The listing builds one solid part. Answer for the finished solid, in the listing's coordinates (mm). A direction names the side the tool comes from. Coordinates: 2 decimals unless noted, no trailing zeros. Order: outer loops, then holes, each group sorted by start corner. A loop starts at its lowest first (then second) coordinate and runs counter-clockwise, first axis right, second up. Notation, with made-up numbers: (74, 81) - (82, 81) arc R13 ccw to (82, 96) - close; hole circle Ø3 at (32.25, 40). An arc over 180 degrees is marked (long way). One line per item, written item: value. Start each with the question number.
```python
from build123d import *

# Parameters (mm, degrees)
SKETCH1_R           = 2
SKETCH1_R_2         = 6
SKETCH1_R_3         = 1.5
BOSS_EXTRUDE1_DEPTH = 3


with BuildPart() as part:
    # Sketch1 → Boss-Extrude1 (new body)
    with BuildSketch(Plane.XY):
        with BuildLine():
            Line((-12.06516619, -3.534722735), (-7.905685951, -9.775614029))
            ThreePointArc((-7.905685951, -9.775614029), (-8.460728899, -12.549046438), (-11.234161307, -11.99400349))
            Line((-11.234161307, -11.99400349), (-11.927408014, -10.953854941))
            ThreePointArc((-11.927408014, -10.953854941), (-12.563289537, -10.527895875), (-13.314124218, -10.676333467))
            Line((-13.314124218, -10.676333467), (-14.001074492, -11.1341777))
            ThreePointArc((-14.001074492, -11.1341777), (-14.438315509, -11.838795077), (-14.193503634, -12.631090792))
            ThreePointArc((-14.193503634, -12.631090792), (15.810257944, 10.537349939), (-17.120545284, -8.239352474))
            ThreePointArc((-17.120545284, -8.239352474), (-16.483484999, -8.770219263), (-15.664866588, -8.637821183))
            Line((-15.664866588, -8.637821183), (-14.977916314, -8.17997695))
            ThreePointArc((-14.977916314, -8.17997695), (-14.551957247, -7.544095427), (-14.70039484, -6.793260745))
            Line((-14.70039484, -6.793260745), (-15.393641546, -5.753112196))
            ThreePointArc((-15.393641546, -5.753112196), (-14.838598598, -2.979679788), (-12.06516619, -3.534722735))
        make_face()
        with Locations((-8.873557843, 13.313901427)):
            Circle(SKETCH1_R, mode=Mode.SUBTRACT)
        with Locations((13.31390139, 8.873557851)):
            Circle(SKETCH1_R, mode=Mode.SUBTRACT)
        with Locations((8.873557814, -13.313901383)):
            Circle(SKETCH1_R, mode=Mode.SUBTRACT)
        Circle(SKETCH1_R_2, mode=Mode.SUBTRACT)
        with Locations((1.668017187, 8.334729669)):
            Circle(SKETCH1_R_3, mode=Mode.SUBTRACT)
        with Locations((-1.668017187, -8.334729669)):
            Circle(SKETCH1_R_3, mode=Mode.SUBTRACT)
        with BuildLine():
            Line((-11.031102319, 3.482424676), (-8.089433024, 2.893712727))
            ThreePointArc((-8.089433024, 2.893712727), (-7.10903413, 1.422720542), (-8.580026315, 0.442321648))
            Line((-8.580026315, 0.442321648), (-11.52169561, 1.031033596))
            ThreePointArc((-11.52169561, 1.031033596), (-12.502094504, 2.502025781), (-11.031102319, 3.482424676))
        make_face(mode=Mode.SUBTRACT)
        with BuildLine():
            Line((11.03081381, -3.483353645), (8.089191886, -2.894405046))
            ThreePointArc((8.089191886, -2.894405046), (7.108911333, -1.423333995), (8.579982384, -0.443053442))
            Line((8.579982384, -0.443053442), (11.521604309, -1.032002041))
            ThreePointArc((11.521604309, -1.032002041), (12.501884862, -2.503073092), (11.03081381, -3.483353645))
        make_face(mode=Mode.SUBTRACT)
    extrude(amount=BOSS_EXTRUDE1_DEPTH)


solid = part.part
```
(1) The part is cut by section A-A on z = 1.8. Count the separate pieces of the cut face and the enclosed holes in it, plus the area to 3 significant figures.
(2) For faces 5 (the face through (-4.5, 4.5, 3)), 6 (the face through (-15.042, -6.28, 1.479)), determine the directions among +Z, -Z, +X, -X, +Y, -Y from which every point of the face is accessible in a straight line to the end or side of a thin tool.
(3) Consider probe 1 along Y at (x, z) = (10.5, 2.5); probe 2 along Y at (x, z) = (12, 2.5); probe 3 along X at (y, z) = (-11.5, 0.5). Determine where each line is inside the solid, lowest interval first.
(4) Flat-ended cylindrical pins translate along their axes: pin 1 Ø3.5 at (x, y) = (1.67, 8.33) entering from +Z; pin 2 Ø1 at (y, z) = (5.5, 2.5) entering from +X; pin 3 Ø3 at (x, y) = (13.31, 8.87) entering from -Z. Find the tip coordinate at first contact, or state that the pin passes through.
(5) The part is cut by section C-C on x = -1. Determine the outline of the cut face in (y, z), plus the area to 3 significant figures.
(6) The part is cut by section B-B on y = -14. Determine the outline of the cut face in (x, z), plus the area to 3 significant figures.
(7) For a pull along Y with two mould halves and no side action, classify faces 1 (the face through (-4.5, 4.5, 0)), 2 (the face through (16.24, 9.86, 1.48)), 3 (the face through (-12.55, -10.53, 1.48)), 4 (the face through (-16.495, -8.767, 1.479)) as pulls with the +Y half, pulls with the -Y half, needs draft (parallel to the pull), parting line crosses it, or undercut.
Completed:
1. separate pieces: 1
1. enclosed holes: 8
1. area: 892 mm2
2. face 5: +Z, +X, -X, +Y, -Y
2. face 6: +Z, -Z
3. probe 1: y = -15.84 to -14.48, -12.15 to -3.38, -0.83 to 15.84
3. probe 2: y = -14.73 to -3.28, -1.24 to 7.37, 10.38 to 14.73
3. probe 3: x = -14.33 to -11.56, -7.67 to 8.03, 9.72 to 15.12
4. pin 1: stops at z = 3
4. pin 2: stops at x = 18.33
4. pin 3: passes through
5. outline: (-18.97, 0) - (-9.68, 0) - (-9.68, 3) - (-18.97, 3) - close; (-6.99, 0) - (-5.92, 0) - (-5.92, 3) - (-6.99, 3) - close; (5.92, 0) - (18.97, 0) - (18.97, 3) - (5.92, 3) - close
5. area: 70.3 mm2
6. outline: (-12.85, 0) - (6.99, 0) - (6.99, 3) - (-12.85, 3) - close; (10.75, 0) - (12.85, 0) - (12.85, 3) - (10.75, 3) - close
6. area: 65.8 mm2
7. face 1: needs draft
7. face 2: parting line crosses it
7. face 3: undercut
7. face 4: pulls with the -Y half
